Verification items for this drawing (mm, ordinates from the low corner). A direction names the side the tool comes from. Round coordinates to 2 decimals unless told otherwise and drop trailing zeros. Loops run counter-clockwise (first coordinate to the right, second up) from the corner with the lowest first, then second, coordinate; pieces in that order, holes last. Notation, with made-up numbers: (80.5, 16) - (109.5, 16) arc R20 cw to (109.5, 47) - close; hole circle Ø9 at (-12, 82). An arc over 180 degrees is marked (long way). Put each result on its own line as item: value.
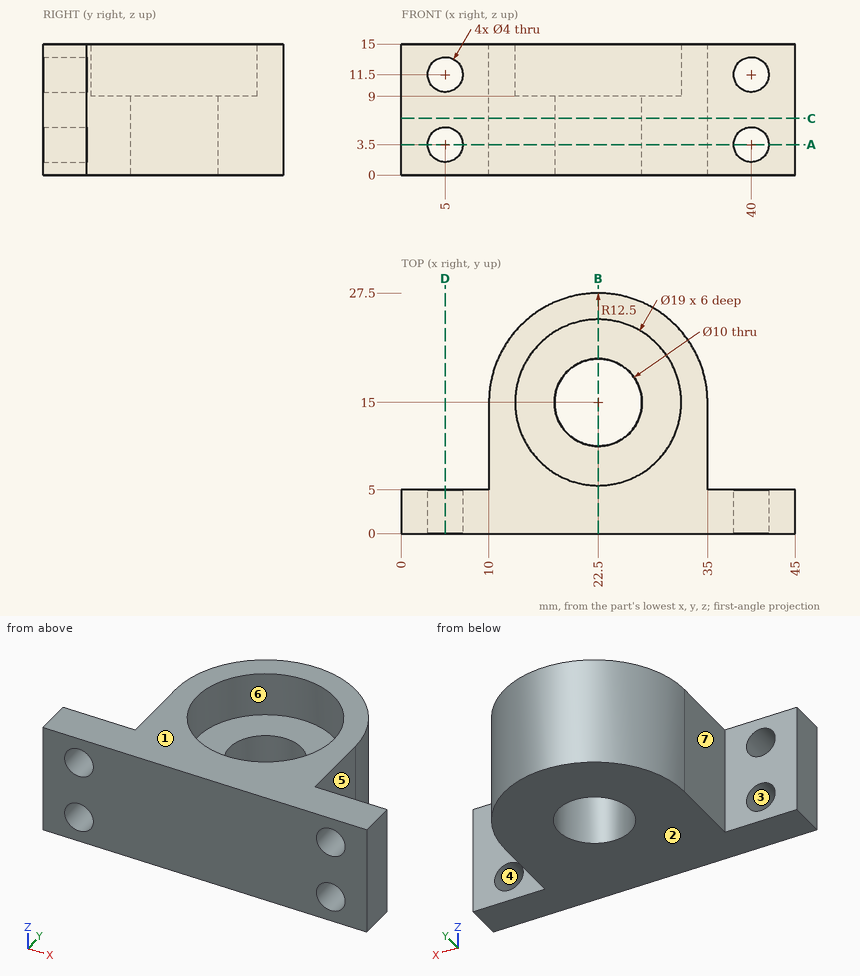
Item 1: Release check for a two-part mould opening along Z. For the marked faces 1, 2, 3 and 4 record: +Z half, -Z half, draft (parallel to the pull), parting line (faces both ways), or undercut.
Filled sheet:
face 1: +Z half
face 2: -Z half
face 3: undercut
face 4: undercut
Item 2: Thickness scan on line 1 (Z direction, x = 40, y = 2.7); line 2 (X direction, y = 1.4, z = 3.5); line 3 (Y direction, x = 22.5, z = 12.4). Record the ranges inside material, lowest first. Write a range as from..to.
Filled sheet:
line 1: 0..1.5, 5.5..9.5, 13.5..15
line 2: 0..3, 7..38, 42..45
line 3: 0..5.5, 24.5..27.5
Item 3: Section check C-C on z = 6.5. Enter the section's corners in (x, y).
Filled sheet:
outline: (0, 0) - (45, 0) - (45, 5) - (35, 5) - (35, 15) arc R12.5 ccw to (10, 15) - (10, 5) - (0, 5) - close; hole circle Ø10 at (22.5, 15)
Item 4: Tool access check on the marked faces 5, 6 and 7. Record the directions out of +Z, -Z, +X, -X, +Y, -Y that give a thin tool (end or side, any length) a straight path to the whole face; none if there is none.
Filled sheet:
face 5: +Z, -Z, +X, +Y
face 6: +Z
face 7: +Z, -Z, -X, +Y
Item 5: Go/stop test with flat-tipped pins: pin 1 (8 mm diameter, centred on x = 4.5, z = 4, fed in from +Y); pin 2 (5 mm diameter, centred on y = 10.5, z = 12, fed in from -X); pin 3 (5 mm diameter, centred on x = 34.5, z = 12, fed in from +Y); pin 4 (8 mm diameter, centred on y = 8.5, z = 7, fed in from -X). Record where each tip stops, or that it passes through.
Filled sheet:
pin 1: y = 5
pin 2: x = 10
pin 3: y = 23.12
pin 4: x = 0
Item 6: Section check B-B on x = 22.5. Enter the section's corners in (y, z), then the cut area to 4 significant figures.
Filled sheet:
outline: (0, 0) - (10, 0) - (10, 9) - (5.5, 9) - (5.5, 15) - (0, 15) - close; (20, 0) - (27.5, 0) - (27.5, 15) - (24.5, 15) - (24.5, 9) - (20, 9) - close
area: 208.5 mm²
Item 7: Section check A-A on z = 3.5. Enter the section's corners in (x, y).
Filled sheet:
outline: (0, 0) - (3, 0) - (3, 5) - (0, 5) - close; (7, 0) - (38, 0) - (38, 5) - (35, 5) - (35, 15) arc R12.5 ccw to (10, 15) - (10, 5) - (7, 5) - close; (42, 0) - (45, 0) - (45, 5) - (42, 5) - close; hole circle Ø10 at (22.5, 15)
Item 8: Section check D-D on x = 5. Enter the section's corners in (y, z), then the cut area to 3 significant figures.
Filled sheet:
outline: (0, 0) - (5, 0) - (5, 1.5) - (0, 1.5) - close; (0, 5.5) - (5, 5.5) - (5, 9.5) - (0, 9.5) - close; (0, 13.5) - (5, 13.5) - (5, 15) - (0, 15) - close
area: 35.0 mm²
